Verification items for the finished model (mm, model axes). Round coordinates to 2 decimals unless told otherwise and drop trailing zeros. Write each loop counter-clockwise with the first axis right and the second up, starting at its lowest first coordinate (ties: lowest second). Pieces come first, ordered by that corner, then holes. Notation, with made-up numbers: M 10,86.5 L 33,86.5 A29 ccw 33,107.5 Z; hole C 88.25,37.5 d1. An arc over 180 degrees is marked long. One line per item, written item: value. Start each with the question number.
Item 1: Thickness scan on probe 1 along Z at (x, y) = (-12, 11); probe 2 along Y at (x, z) = (-40, 3); probe 3 along Y at (x, z) = (-5.5, -27). Record the ranges inside material, lowest first. Write a range as from..to.
Item 2: Gauge pin test, flat ends, axial feed: pin 1 (1.5 mm diameter, centred on x = -17.5, y = 13, fed in from -Z); pin 2 (12 mm diameter, centred on x = -16, y = 14.5, fed in from -Z); pin 3 (3 mm diameter, centred on y = 3, z = 31.5, fed in from -X); pin 4 (3.5 mm diameter, centred on x = -3.5, z = 0, fed in from +Y). Record the tip position at first contact, or that the pin passes through.
Item 3: Section check B-B, the plane z = 0. Record the cut outline in (x, y).
Item 4: Section check C-C, the plane x = -22.5. Record the cut outline in (y, z).
Item 5: Section check D-D, the plane x = 0. Record the cut outline in (y, z).
Item 6: Section check A-A, the plane y = 13.25. Record the cut outline in (x, z).
from build123d import *

# Parameters (mm, degrees)
SKETCH1_R           = 50
BOSS_EXTRUDE1_DEPTH = 5
SKETCH2_R           = 15
BOSS_EXTRUDE2_DEPTH = 5
BOSS_EXTRUDE3_DEPTH = 5
CUT_EXTRUDE1_DEPTH  = 5
SKETCH6_R           = 2.088892153
BOSS_EXTRUDE4_DEPTH = 10


with BuildPart() as part:
    # Sketch1 → Boss-Extrude1 (new body)
    with BuildSketch(Plane(origin=(0, 0, 0), x_dir=(1, 0, 0), z_dir=(0, 1, 0))):
        with Locations(Location((0, 0, 0), (0, 0, 270))):
            Circle(SKETCH1_R)
    extrude(amount=BOSS_EXTRUDE1_DEPTH)

    # Sketch2 → Boss-Extrude2 (add)
    with BuildSketch(Plane(origin=(0, 5, 0), x_dir=(1, 0, 0), z_dir=(0, 1, 0))):
        with Locations(Location((0, 0, 0), (0, 0, 270))):
            Circle(SKETCH2_R)
    extrude(amount=BOSS_EXTRUDE2_DEPTH)

    # Sketch4 → Boss-Extrude3 (add)
    with BuildSketch(Plane(origin=(0, 10, 0), x_dir=(1, 0, 0), z_dir=(0, 1, 0))):
        with BuildLine():
            Line((9.847634435, -4.252387597), (-44.314354955, -4.252387597))
            ThreePointArc((-44.314354955, -4.252387597), (-48.566742552, 0), (-44.314354955, 4.252387597))
            Line((-44.314354955, 4.252387597), (9.847634435, 4.252387597))
            ThreePointArc((9.847634435, 4.252387597), (14.100022031, 0), (9.847634435, -4.252387597))
        make_face()
    extrude(amount=BOSS_EXTRUDE3_DEPTH)

    # Sketch5 → Cut-Extrude1 (cut)
    with BuildSketch(Plane(origin=(0, 15, 0), x_dir=(1, 0, 0), z_dir=(0, 1, 0))):
        with BuildLine():
            Line((5.222230382, -2.312702026), (-44.314354955, -2.312702026))
            ThreePointArc((-44.314354955, -2.312702026), (-46.627056982, 0), (-44.314354955, 2.312702026))
            Line((-44.314354955, 2.312702026), (5.222230382, 2.312702026))
            ThreePointArc((5.222230382, 2.312702026), (7.534932408, 0), (5.222230382, -2.312702026))
        make_face()
    extrude(amount=-CUT_EXTRUDE1_DEPTH, mode=Mode.SUBTRACT)

    # Sketch6 → Boss-Extrude4 (add)
    with BuildSketch(Plane(origin=(0, 10, 0), x_dir=(1, 0, 0), z_dir=(0, 1, 0))):
        with Locations(Location((0, 0, 0), (0, 0, 270))):
            Circle(SKETCH6_R)
    extrude(amount=BOSS_EXTRUDE4_DEPTH)


solid = part.part
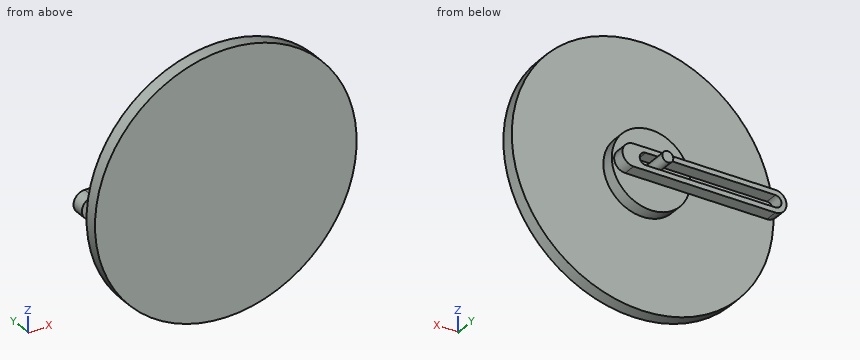
Response values:
1. probe 1: z = -4.25..-2.31, 2.31..4.25
1. probe 2: y = 0..5, 10..15
1. probe 3: y = 0..5
2. pin 1: stops at z = -4.25
2. pin 2: stops at z = -8.96
2. pin 3: stops at x = -40
2. pin 4: stops at y = 20
3. outline: M -50,0 L 50,0 L 50,5 L 15,5 L 15,10 L 14.1,10 L 14.1,15 L 7.53,15 L 7.53,10 L 2.09,10 L 2.09,20 L -2.09,20 L -2.09,10 L -15,10 L -15,5 L -50,5 Z; M -48.57,10 L -46.63,10 L -46.63,15 L -48.57,15 Z
4. outline: M 0,-44.65 L 5,-44.65 L 5,44.65 L 0,44.65 Z; M 10,-4.25 L 15,-4.25 L 15,-2.31 L 10,-2.31 Z; M 10,2.31 L 15,2.31 L 15,4.25 L 10,4.25 Z
5. outline: M 0,-50 L 5,-50 L 5,-15 L 10,-15 L 10,-4.25 L 15,-4.25 L 15,-2.31 L 10,-2.31 L 10,-2.09 L 20,-2.09 L 20,2.09 L 10,2.09 L 10,2.31 L 15,2.31 L 15,4.25 L 10,4.25 L 10,15 L 5,15 L 5,50 L 0,50 Z
6. outline: M -44.31,-4.25 L 9.85,-4.25 A4.25 ccw 9.85,4.25 L -44.31,4.25 A4.25 ccw Z; C 0,0 d4.18; hole M -44.31,-2.31 L 5.22,-2.31 A2.31 ccw 5.22,2.31 L -44.31,2.31 A2.31 ccw Z
